Build history of the part. All positions in model axes, mm. A direction names the side the tool comes from. Coordinates: 2 decimals unless noted, no trailing zeros. Loops run counter-clockwise (first coordinate to the right, second up) from the corner with the lowest first, then second, coordinate; pieces in that order, holes last.
(1) Slice it at D-D (y = -3.5). Give the cut face in (x, z).
(2) Slice it at C-C (x = -37). Give the cut face in (y, z).
(3) Flat gauge pins, fed straight in: P1, Ø6, axis at x = 38, y = -18.5, coming from the -Z side; P2, Ø7.5, axis at x = -9.5, y = -13, coming from the +Z side; P3, Ø5.5, axis at y = -13.5, z = -15.5, coming from the +X side. Where does each tip first touch, or does it go through?
(4) Slice it at B-B (y = -16). Give the cut face in (x, z), and give its area (3 significant figures).
(5) Tool access for faces 5 (the face through (50.8, -13, 13)), 6 (the face through (41, -6, -6.317)), 7 (the face through (25.4, -13, 19)): list every direction of +Z, -Z, +X, -X, +Y, -Y with a clear straight run to the whole face (end or side of a thin tool).
(6) Slice it at A-A (z = 0). Give the cut face in (x, y).
(7) Two-plate mould, pull along X, no slides. Class faces 1 (the face through (0, -13, 12.7)), 2 (the face through (31.75, -13, -16)), 3 (the face through (-50.8, -15.3, -6)), 4 (the face through (-10, -13, -25.4)): pulls with the +X half, pulls with the -X half, needs draft (parallel to the pull), parting line crosses it, or undercut.
(8) Wall check: L1, parallel to Z at x = 2, y = -12.7; L2, parallel to X at y = -7.75, z = 13; L3, parallel to Y at x = 19, z = 0. Give the ranges that are in metal, low to high.
from build123d import *

# Parameters (mm, degrees)
F0_W     = 101.6
F0_H     = 50.8
F1_DEPTH = 25.4
F2_W     = 25.4
F2_H     = 19.083421053
F3_DEPTH = 19.05
F4_W     = 50.8
F4_H     = 25.4
F5_DEPTH = 12.7
F6_R     = 6.35
F7_DEPTH = 101.601


with BuildPart() as f1:
    # F0 (on Front) → F1 (new body)
    with BuildSketch(Plane.XZ):
        Rectangle(F0_W, F0_H)
    extrude(amount=F1_DEPTH)

    # F2 (on face) → F3 (cut)
    with BuildSketch(Plane.YZ.offset(50.8)):
        with Locations((-12.7, -15.8582894735)):
            Rectangle(F2_W, F2_H)
    extrude(amount=-F3_DEPTH, mode=Mode.SUBTRACT)

    # F4 (on face) → F5 (cut)
    with BuildSketch(Plane.XY.offset(25.4)):
        with Locations((0, -12.7)):
            Rectangle(F4_W, F4_H)
    extrude(amount=-F5_DEPTH, mode=Mode.SUBTRACT)

    # F6 (on face) → F7 (cut, through all)
    with BuildSketch(Plane.YZ.offset(50.8)):
        with Locations((-12.7, 0)):
            Circle(F6_R)
    extrude(amount=-F7_DEPTH, mode=Mode.SUBTRACT)


solid = f1.part
Response values:
1. outline: (-50.8, -25.4) - (31.75, -25.4) - (31.75, -6.32) - (50.8, -6.32) - (50.8, 25.4) - (25.4, 25.4) - (25.4, 12.7) - (-25.4, 12.7) - (-25.4, 25.4) - (-50.8, 25.4) - close
2. outline: (-25.4, -25.4) - (0, -25.4) - (0, 25.4) - (-25.4, 25.4) - close; hole circle Ø12.7 at (-12.7, 0)
3. P1: stops at z = -6.32
3. P2: stops at z = 12.7
3. P3: stops at x = 31.75
4. outline: (-50.8, -25.4) - (31.75, -25.4) - (31.75, -6.32) - (50.8, -6.32) - (50.8, -5.43) - (-50.8, -5.43) - close; (-50.8, 5.43) - (50.8, 5.43) - (50.8, 25.4) - (25.4, 25.4) - (25.4, 12.7) - (-25.4, 12.7) - (-25.4, 25.4) - (-50.8, 25.4) - close
4. area: 3,050 mm2
5. face 5: +Z, -Z, +X, +Y, -Y
5. face 6: -Z, +X, +Y, -Y
5. face 7: +Z, +Y, -Y
6. outline: (-50.8, -25.4) - (50.8, -25.4) - (50.8, -19.05) - (-50.8, -19.05) - close; (-50.8, -6.35) - (50.8, -6.35) - (50.8, 0) - (-50.8, 0) - close
7. face 1: undercut
7. face 2: pulls with the +X half
7. face 3: pulls with the -X half
7. face 4: needs draft
8. L1: z = -25.4 to -6.35, 6.35 to 12.7
8. L2: x = -50.8 to -25.4, 25.4 to 50.8
8. L3: y = -25.4 to -19.05, -6.35 to 0
